```python
from build123d import *
from build123d.topology import SkipClean

# Parameters (mm, degrees)
SKETCH1_W                        = 91
SKETCH1_H                        = 133
BOSS_EXTRUDE1_DEPTH              = 9
SKETCH8_W                        = 85.75
SKETCH8_H                        = 121
BOSS_EXTRUDE2_DEPTH              = 8
F_1_8_0_125_DIAMETER_HOLE1_D     = 3.175
F_1_8_0_125_DIAMETER_HOLE1_DEPTH = 15.439
F_1_8_0_125_DIAMETER_HOLE1_TIP   = 0.953866233
CUT_EXTRUDE1_DEPTH               = 83.349863388
CUT_EXTRUDE1_DEPTH_BACK          = 83.349863388
SKETCH9_W                        = 35
SKETCH9_H                        = 8
CUT_EXTRUDE2_DEPTH               = 83.349863388
TAP_DRILL_FOR_10_32_TAP1_D       = 4.0386
TAP_DRILL_FOR_10_32_TAP1_DEPTH   = 6
F_10_CLEARANCE_HOLE1_D           = 4.9784
F_10_CLEARANCE_HOLE1_DEPTH       = 6
TAP_DRILL_FOR_4_40_TAP1_REACH    = 84.35
TAP_DRILL_FOR_4_40_TAP1_BORE_R   = 1.1303
TAP_DRILL_FOR_6_32_TAP1_D        = 2.7051
CUT_EXTRUDE4_REACH               = 143.592
SKETCH20_W                       = 9.5
SKETCH20_H                       = 9
CUT_EXTRUDE5_DEPTH               = 81.929077829
CUT_EXTRUDE5_DEPTH_BACK          = 81.929077829
SKETCH21_OUTSIDE_W               = 119.582
SKETCH21_OUTSIDE_H               = 166.832
SKETCH21_OUTSIDE_W_2             = 72
SKETCH21_OUTSIDE_H_2             = 133
SKETCH22_W                       = 11.4873
SKETCH22_H                       = 121
SKETCH22_R                       = 1.5875
BOSS_EXTRUDE3_DEPTH              = 8


with BuildPart() as part:
    # Sketch1 → Boss-Extrude1 (new body)
    with BuildSketch(Plane(origin=(0, 0, 0), x_dir=(1, 0, 0), z_dir=(0, 1, 0))):
        Rectangle(SKETCH1_W, SKETCH1_H)
    extrude(amount=-BOSS_EXTRUDE1_DEPTH)

    # Sketch8 → Boss-Extrude2 (add)
    with BuildSketch(Plane.XZ.offset(9)):
        Rectangle(SKETCH8_W, SKETCH8_H)
    extrude(amount=BOSS_EXTRUDE2_DEPTH)

    # 1/8 (0.125) Diameter Hole1
    with Locations(Plane(origin=(0, -17, 0), x_dir=(-1, 0, 0), z_dir=(0, -1, 0))):
        with Locations((-12.7, -38.1), (-12.7, 38.1)):
            Hole(F_1_8_0_125_DIAMETER_HOLE1_D / 2, depth=F_1_8_0_125_DIAMETER_HOLE1_DEPTH)
            with Locations((0, 0, -(F_1_8_0_125_DIAMETER_HOLE1_DEPTH + F_1_8_0_125_DIAMETER_HOLE1_TIP / 2))):  # 118° drill point
                Cone(0, F_1_8_0_125_DIAMETER_HOLE1_D / 2, F_1_8_0_125_DIAMETER_HOLE1_TIP, mode=Mode.SUBTRACT)

    # Sketch9 → Cut-Extrude1 (cut, two sides: drawn at the far end of the back side and taken through both)
    with BuildSketch(Plane.XY.offset(-CUT_EXTRUDE1_DEPTH_BACK)):
        with Locations((0, -13)):
            Rectangle(SKETCH9_W, SKETCH9_H)
    extrude(amount=CUT_EXTRUDE1_DEPTH + CUT_EXTRUDE1_DEPTH_BACK, mode=Mode.SUBTRACT)

    # Sketch10 → Cut-Extrude2 (cut, through all)
    with BuildSketch(Plane(origin=(0, 0, 0), x_dir=(1, 0, 0), z_dir=(0, 1, 0))):
        Polygon((-6, 60.5), (6, 60.5), (6.0127, 60.5), (6.0127, -60.5), (6, -60.5), (-6, -60.5), (-9, -60.5), (-9, 60.5), align=None)
    extrude(amount=-CUT_EXTRUDE2_DEPTH, mode=Mode.SUBTRACT)

    # Tap Drill for #10-32 Tap1
    with Locations(Plane.XY.offset(-60.5)):
        with Locations((0, -6)):
            Hole(TAP_DRILL_FOR_10_32_TAP1_D / 2, depth=TAP_DRILL_FOR_10_32_TAP1_DEPTH)

    # #10 Clearance Hole1
    with Locations(Plane.XY.offset(66.5)):
        with Locations((0, -6)):
            Hole(F_10_CLEARANCE_HOLE1_D / 2, depth=F_10_CLEARANCE_HOLE1_DEPTH)

    # Tap Drill for #4-40 Tap1 bore → Tap Drill for #4-40 Tap1 (cut, up to next)
    with BuildSketch(Plane(origin=(0, 0, 0), x_dir=(1, 0, 0), z_dir=(0, 1, 0)), mode=Mode.PRIVATE) as tap_drill_for_4_40_tap1_sk1:
        with Locations((0, -63.5)):
            Circle(TAP_DRILL_FOR_4_40_TAP1_BORE_R)
    tap_drill_for_4_40_tap1_tool1 = extrude(tap_drill_for_4_40_tap1_sk1.sketch, amount=-TAP_DRILL_FOR_4_40_TAP1_REACH, mode=Mode.PRIVATE) & part.part
    add(tap_drill_for_4_40_tap1_tool1.solids().sort_by_distance((0, 0, 63.5))[0], mode=Mode.SUBTRACT)

    # Tap Drill for #6-32 Tap1 (through all)
    with Locations(Plane(origin=(0, 0, 0), x_dir=(1, 0, 0), z_dir=(0, 1, 0))):
        with Locations((-18, -63.5), (18, -63.5), (18, 63.5), (-18, 63.5)):
            Hole(TAP_DRILL_FOR_6_32_TAP1_D / 2)

    # Sketch20 → Cut-Extrude4 (cut, up to next)
    with BuildSketch(Plane.XY.offset(66.5), mode=Mode.PRIVATE) as cut_extrude4_sk1:
        with Locations((40.75, -4.5)):
            Rectangle(SKETCH20_W, SKETCH20_H)
    cut_extrude4_tool1 = extrude(cut_extrude4_sk1.sketch, amount=-CUT_EXTRUDE4_REACH, mode=Mode.PRIVATE) & part.part
    # Sketch20 → Cut-Extrude4 (cut, up to next)
    with BuildSketch(Plane.XY.offset(66.5), mode=Mode.PRIVATE) as cut_extrude4_sk2:
        with Locations((-40.75, -4.5)):
            Rectangle(SKETCH20_W, SKETCH20_H)
    cut_extrude4_tool2 = extrude(cut_extrude4_sk2.sketch, amount=-CUT_EXTRUDE4_REACH, mode=Mode.PRIVATE) & part.part
    add(cut_extrude4_tool1.solids().sort_by_distance((40.75, -4.5, 66.5))[0], mode=Mode.SUBTRACT)
    add(cut_extrude4_tool2.solids().sort_by_distance((-40.75, -4.5, 66.5))[0], mode=Mode.SUBTRACT)

    # Sketch21 outside → Cut-Extrude5 (cut, two sides: drawn at the far end of the back side and taken through both)
    with BuildSketch(Plane(origin=(0, 0, 0), x_dir=(1, 0, 0), z_dir=(0, 1, 0)).offset(-CUT_EXTRUDE5_DEPTH_BACK)):
        Rectangle(SKETCH21_OUTSIDE_W, SKETCH21_OUTSIDE_H)
        Rectangle(SKETCH21_OUTSIDE_W_2, SKETCH21_OUTSIDE_H_2, mode=Mode.SUBTRACT)
    extrude(amount=CUT_EXTRUDE5_DEPTH + CUT_EXTRUDE5_DEPTH_BACK, mode=Mode.SUBTRACT)

    # Sketch22 → Boss-Extrude3 (add)
    with SkipClean():  # the faces are left unmerged after this step: merging them gives an invalid solid
        with BuildSketch(Plane.XZ.offset(9)):
            with Locations((11.75635, 0)):
                Rectangle(SKETCH22_W, SKETCH22_H)
            with Locations(Location((12.7, 38.1, 0), (0, 0, 270))):
                Circle(SKETCH22_R, mode=Mode.SUBTRACT)
            with Locations(Location((12.7, -38.1, 0), (0, 0, 270))):
                Circle(SKETCH22_R, mode=Mode.SUBTRACT)
        extrude(amount=BOSS_EXTRUDE3_DEPTH)


solid = part.part
```
Design review of the part built by this model. Coordinates are the model's own, in mm. A direction names the side the tool comes from. Round coordinates to 2 decimals unless told otherwise and drop trailing zeros. Write each loop counter-clockwise with the first axis right and the second up, starting at its lowest first coordinate (ties: lowest second). Pieces come first, ordered by that corner, then holes.
Item 1: Clearance check with flat-ended pins moving along their axes: pin 1 Ø6.5 at (x, y) = (-26.5, -14) entering from +Z; pin 2 Ø9 at (x, y) = (23, -12) entering from -Z; pin 3 Ø9 at (x, y) = (12.5, -14) entering from -Z. State where each tip first meets the part, or that it passes through.
Item 2: We need section D-D on y = -6. Write out the cut boundary in (x, z) (1 decimal), and give its area (3 significant figures).
Item 3: We need section C-C on x = 4. Write out the cut boundary in (y, z), and give its area (3 significant figures).
Item 4: For probe 1 along X at (y, z) = (-5.75, 38.1); probe 2 along Z at (x, y) = (-18, -5.5); probe 3 along X at (y, z) = (-5.75, 63.5), list the stretches that pass through material, from the lowest coordinate up.
Item 5: The part is to be moulded in two halves that separate along Z. For faces 1 (the flat face through (-9, -4, 1)), 2 (the flat face through (-1, -3, -66.5)), 3 (the flat face through (7, 0, -1)), 4 (the flat face through (-1, -4, -60.5)), say which applies: +Z half, -Z half, draft (parallel to the pull), parting line (faces both ways), or undercut.
Item 6: We need section A-A on z = -63.5. Write out the cut boundary in (x, y), and give its area (3 significant figures).
Item 7: For faces 5 (the flat face through (-17.5, -13, -1)), 6 (the flat face through (-27, -13, 60.5)), 7 (the cylindrical face through (-1.149, -8.208, 63.458)), 8 (the flat face through (-27, -13, -60.5)), 9 (the flat face through (-2, -3, 60.5)), list the 3-axis set-ups (+Z, -Z, +X, -X, +Y, -Y) from which the entire face can be reached by the end or side of a thin tool; tool diameter is ignored.
Returned:
1. pin 1: stops at z = 60.5
1. pin 2: stops at z = -66.5
1. pin 3: stops at z = -60.5
2. outline: (-36, -66.5) - (-2, -66.5) - (-2, -60.5) - (-9, -60.5) - (-9, 60.5) - (-2.5, 60.5) - (-2.5, 66.5) - (-36, 66.5) - close; (2, -66.5) - (36, -66.5) - (36, 66.5) - (2.5, 66.5) - (2.5, 60.5) - (6, 60.5) - (6, -60.5) - (2, -60.5) - close; hole circle Ø2.7 at (-18, -63.5); hole circle Ø2.7 at (-18, 63.5); hole circle Ø3.2 at (12.7, -38.1); hole circle Ø3.2 at (12.7, 38.1); hole circle Ø2.7 at (18, -63.5); hole circle Ø2.7 at (18, 63.5)
2. area: 7,670 mm2
3. outline: (-9, -66.5) - (0, -66.5) - (0, -60.5) - (-9, -60.5) - close; (-9, 60.5) - (0, 60.5) - (0, 66.5) - (-9, 66.5) - close
3. area: 108 mm2
4. probe 1: x = -36 to -9, 6.01 to 11.11, 14.29 to 36
4. probe 2: z = -66.5 to -64.85, -62.15 to 62.15, 64.85 to 66.5
4. probe 3: x = -36 to -19.35, -16.65 to -2.48, 2.48 to 16.65, 19.35 to 36
5. face 1: undercut
5. face 2: -Z half
5. face 3: draft
5. face 4: undercut
6. outline: (-36, -9) - (-19.35, -9) - (-19.35, 0) - (-36, 0) - close; (-16.65, -9) - (16.65, -9) - (16.65, 0) - (-16.65, 0) - close; (19.35, -9) - (36, -9) - (36, 0) - (19.35, 0) - close; hole circle Ø4.04 at (0, -6)
6. area: 586 mm2
7. face 5: +Z, -Z, -Y
7. face 6: +Z, +X, -X, -Y
7. face 7: +Z
7. face 8: -Z, +X, -X, -Y
7. face 9: +Y, -Y
